The model under review builds one solid part; all positions refer to its coordinate system, in mm. Round coordinates to 2 decimals unless told otherwise and drop trailing zeros. Loops run counter-clockwise (first coordinate to the right, second up) from the corner with the lowest first, then second, coordinate; pieces in that order, holes last. Notation, with made-up numbers: (-29, 88) - (4, 88) arc R30 cw to (4, 117) - close; hole circle Ø3 at (-35, 26.25). An arc over 180 degrees is marked (long way). Answer as CSV lines item,"result".
from build123d import *

# Parameters (mm, degrees)
F1_DEPTH = 20
F2_R     = 300
F3_DEPTH = 20.001
F4_R     = 5


with BuildPart() as f1:
    # F0 (on Top) → F1 (new body)
    with BuildSketch(Plane.XY):
        Polygon((70, 0), (-70, 0), (-70, -100), (-200, -100), (-200, -600), (200, -600), (200, -100), (70, -100), align=None)
    extrude(amount=F1_DEPTH)

    # F2 (on face) → F3 (intersect, through all)
    with BuildSketch(Plane.XY.offset(20)):
        with Locations((0, -280)):
            Circle(F2_R)
    extrude(amount=-F3_DEPTH, mode=Mode.INTERSECT)

    # F4
    f4_edges = [f1.edges().sort_by_distance(p)[0] for p in [
        (70, -50, 20),
        (135, -100, 20),
        (200, -301.803399, 20),
        (0, -580, 20),
        (-200, -301.803399, 20),
        (-135, -100, 20),
        (-70, -50, 20),
        (0, 0, 20),
        (70, 0, 10),
        (-70, 0, 10),
        (0, 0, 0),
        (70, -50, 0),
        (135, -100, 0),
        (200, -301.803399, 0),
        (0, -580, 0),
        (-200, -301.803399, 0),
        (-135, -100, 0),
        (-70, -50, 0),
        (200, -100, 10),
        (70, -100, 10),
        (-70, -100, 10),
        (-200, -100, 10),
        (200, -503.606798, 10),
        (-200, -503.606798, 10),
    ]]
    fillet(f4_edges, radius=F4_R)


solid = f1.part
1. Take a section at A-A (z = 9). State the section outline as (x, y) points, plus the area to 3 significant figures.
Numbers:
outline,"(-200, -501.36) arc R5 ccw to (-198.31, -505.11) arc R300 ccw to (198.31, -505.11) arc R5 ccw to (200, -501.36) - (200, -105) arc R5 ccw to (195, -100) - (75, -100) arc R5 cw to (70, -95) - (70, -5) arc R5 ccw to (65, 0) - (-65, 0) arc R5 ccw to (-70, -5) - (-70, -95) arc R5 cw to (-75, -100) - (-195, -100) arc R5 ccw to (-200, -105) - close"
area,"196,000 mm²"
2. Clearance check with flat-ended pins moving along their axes: pin 1 (1.5 mm diameter, centred on y = -243, z = 4, fed in from +X); pin 2 (1.5 mm diameter, centred on x = 156, z = 8, fed in from +Y); pin 3 (12 mm diameter, centred on y = -85.5, z = 5.5, fed in from +X). State where each tip first meets the part, or that it passes through.
Numbers:
pin 1,"stops at x = 199.99"
pin 2,"stops at y = -100"
pin 3,"stops at x = 70"
3. Wall thickness on probe 1 along X at (y, z) = (-36.5, 5.25); probe 2 along Y at (x, z) = (-8, 11.25); probe 3 along Y at (x, z) = (4, 10.25): over which ranges is each line inside the solid? List them lowest first.
Numbers:
probe 1,"x = -70 to 70"
probe 2,"y = -579.89 to 0"
probe 3,"y = -579.97 to 0"
